```python
from build123d import *

# Parameters (mm, degrees)
SKETCH_W     = 100
SKETCH_H     = 75
PAD_DEPTH    = 10
SKETCH001_W  = 25
SKETCH001_H  = 75
PAD001_DEPTH = 10
SKETCH002_W  = 25
SKETCH002_H  = 75
PAD002_DEPTH = 10


with BuildPart() as part:
    # Sketch → Pad (new body)
    with BuildSketch(Plane.XY):
        with Locations((50, 37.5)):
            Rectangle(SKETCH_W, SKETCH_H)
    extrude(amount=PAD_DEPTH)

    # Sketch001 → Pad001 (new body)
    with BuildSketch(Plane.XY.offset(10)):
        with Locations((50, 37.5)):
            Rectangle(SKETCH001_W, SKETCH001_H)
    extrude(amount=PAD001_DEPTH)

    # Sketch002 → Pad002 (new body)
    with BuildSketch(Plane(origin=(0, 0, 0), x_dir=(1, 0, 0), z_dir=(0, 0, -1))):
        with Locations((50, -37.5)):
            Rectangle(SKETCH002_W, SKETCH002_H)
    extrude(amount=PAD002_DEPTH)


solid = part.part
```
Geometry check sheet. Reference: the model listing, model coordinates, mm. A direction names the side the tool comes from. Round coordinates to 2 decimals unless told otherwise and drop trailing zeros. Loops run counter-clockwise (first coordinate to the right, second up) from the corner with the lowest first, then second, coordinate; pieces in that order, holes last. Notation, with made-up numbers: (65.5, 44) - (69.5, 44) arc R31 cw to (69.5, 79) - close; hole circle Ø4 at (-14.5, 6.25). An arc over 180 degrees is marked (long way). Use a Markdown table: item, result.
Q1. Cross-section at A-A on y = 44.5. Record the cut outline in (x, z), plus the area to 3 significant figures.
Solutions:
| item | result |
|---|---|
| outline | (0, 0) - (37.5, 0) - (37.5, -10) - (62.5, -10) - (62.5, 0) - (100, 0) - (100, 10) - (62.5, 10) - (62.5, 20) - (37.5, 20) - (37.5, 10) - (0, 10) - close |
| area | 1,500 mm2 |
Q2. Cross-section at B-B on z = -1.5. Record the cut outline in (x, y), plus the area to 4 significant figures.
Solutions:
| item | result |
|---|---|
| outline | (37.5, 0) - (62.5, 0) - (62.5, 75) - (37.5, 75) - close |
| area | 1,875 mm2 |
Q3. Material ranges on line 1 (Z direction, x = 78, y = 12.5); line 2 (X direction, y = 7.5, z = -0.75), recorded low to high.
Solutions:
| item | result |
|---|---|
| line 1 | z = 0 to 10 |
| line 2 | x = 37.5 to 62.5 |
Q4. Access from +Z, -Z, +X, -X, +Y, -Y to the whole of each face (thin tool, end or side, straight path). Record for faces 1 (the flat face through (37.5, 38, -5)), 2 (the flat face through (62.5, 38, -5)), 3 (the flat face through (37.5, 37, 15)).
Solutions:
| item | result |
|---|---|
| face 1 | -Z, -X, +Y, -Y |
| face 2 | -Z, +X, +Y, -Y |
| face 3 | +Z, -X, +Y, -Y |
Q5. Cross-section at C-C on x = 24.5. Record the cut outline in (y, z), plus the area to 3 significant figures.
Solutions:
| item | result |
|---|---|
| outline | (0, 0) - (75, 0) - (75, 10) - (0, 10) - close |
| area | 750 mm2 |
Q6. Go/stop test with flat-tipped pins: P1, Ø12, axis at x = 89, y = 23.5, coming from the +Z side; P2, Ø3, axis at y = 21.5, z = -3, coming from the -X side; P3, Ø5, axis at y = 29.5, z = -4, coming from the +X side. Record where each tip stops, or that it passes through.
Solutions:
| item | result |
|---|---|
| P1 | stops at z = 10 |
| P2 | stops at x = 37.5 |
| P3 | stops at x = 62.5 |
